```python
from build123d import *


with BuildPart() as f1:
    # F0 (on Front) → F1 (revolve)
    with BuildSketch(Plane.XZ):
        with BuildLine():
            Line((-6.821418, 16.058695), (0, 16.058695))
            Line((0, 16.058695), (0, 18.716853))
            Line((0, 18.716853), (-5.596306, 18.716853))
            ThreePointArc((-5.596306, 18.716853), (-7.781779, 19.457771), (-9.066084, 21.375012))
            Line((-9.066084, 21.375012), (-11.192611, 21.375012))
            Line((-11.192611, 21.375012), (-11.192611, 14.40473))
            Line((-11.192611, 14.40473), (-9.302366, 14.40473))
            Line((-9.302366, 14.40473), (-9.302366, 12.750765))
            Line((-9.302366, 12.750765), (-11.192611, 12.750765))
            Line((-11.192611, 12.750765), (-11.192611, 10.687506))
            Line((-11.192611, 10.687506), (-9.302366, 10.687506))
            Line((-9.302366, 10.687506), (-9.302366, 9.442835))
            Line((-9.302366, 9.442835), (-11.192611, 9.442835))
            Line((-11.192611, 9.442835), (-11.192611, 7.316309))
            Line((-11.192611, 7.316309), (-9.302366, 7.316309))
            Line((-9.302366, 7.316309), (-9.302366, 6.253046))
            Line((-9.302366, 6.253046), (-11.192611, 6.253046))
            Line((-11.192611, 6.253046), (-11.192611, 0))
            Line((-11.192611, 0), (-6.821418, 0))
            Line((-6.821418, 0), (-6.821418, 16.058695))
        make_face()
    revolve(axis=Axis((0, 0, 17.387774), (0, 0, -1)))


solid = f1.part
```
Model file for the job. Use its own axes, mm. A direction names the side the tool comes from. Round coordinates to 2 decimals unless told otherwise and drop trailing zeros. Write each loop counter-clockwise with the first axis right and the second up, starting at its lowest first coordinate (ties: lowest second). Pieces come first, ordered by that corner, then holes. Notation, with made-up numbers: (10.25, 29.5) - (42.25, 29.5) arc R34 ccw to (42.25, 61.5) - close; hole circle Ø7 at (84, 72.25). An arc over 180 degrees is marked (long way). Use CSV: the item, a comma, the result in double quotes. Start each with the question number.
Item 1: Band-saw the part on B-B (z = 4.75). Write the cut outline in (x, y).
Item 2: Drill centre lines: L1, parallel to Z at x = -5.5, y = -7.75; L2, parallel to Y at x = 0, z = 12.5; L3, parallel to Y at x = 1.5, z = 3.25. Where is each one in solid material? Low to high. Write a range as [from, to].
Item 3: Two-plate mould, pull along X, no slides. Class faces 1 (the face through (-8.873, 2.794, 13.566)), 2 (the face through (0, 0, 18.717)), 3 (the face through (0, 0, 16.059)), 4 (the face through (3, 9, 14.405)): released by +X, released by -X, zero draft, split by the parting line, or undercut.
Item 4: Band-saw the part on A-A (z = 17). Write the cut outline in (x, y).
Item 5: Tool access for faces 5 (the face through (-6.506, 2.049, 8.142)), 6 (the face through (-10.676, 3.362, 3.083)), 7 (the face through (3, 9, 7.316)): list every direction of +Z, -Z, +X, -X, +Y, -Y with a clear straight run to the whole face (end or side of a thin tool).
Item 6: Pin check, flat tips, straight feed: P1, Ø4, axis at x = -1.5, y = 0.5, coming from the -Z side; P2, Ø4, axis at x = 5.5, z = 18, coming from the -Y side; P3, Ø1, axis at y = 6, z = 12.5, coming from the +X side. Stop position of each tip, or through.
Checked values:
1,outline,"circle Ø22.39 at (0, 0); hole circle Ø13.64 at (0, 0)"
2,L1,"z = [0, 6.25], [7.32, 9.44], [10.69, 12.75], [14.4, 21.38]"
2,L2,"y = [-11.19, -6.82], [6.82, 11.19]"
2,L3,"y = [-11.09, -6.65], [6.65, 11.09]"
3,face 1,"split by the parting line"
3,face 2,"undercut"
3,face 3,"undercut"
3,face 4,"zero draft"
4,outline,"circle Ø22.39 at (0, 0)"
5,face 5,"-Z"
5,face 6,"+Z, -Z"
5,face 7,"none"
6,P1,"stops at z = 16.06"
6,P2,"stops at y = -10.63"
6,P3,"stops at x = 9.75"
